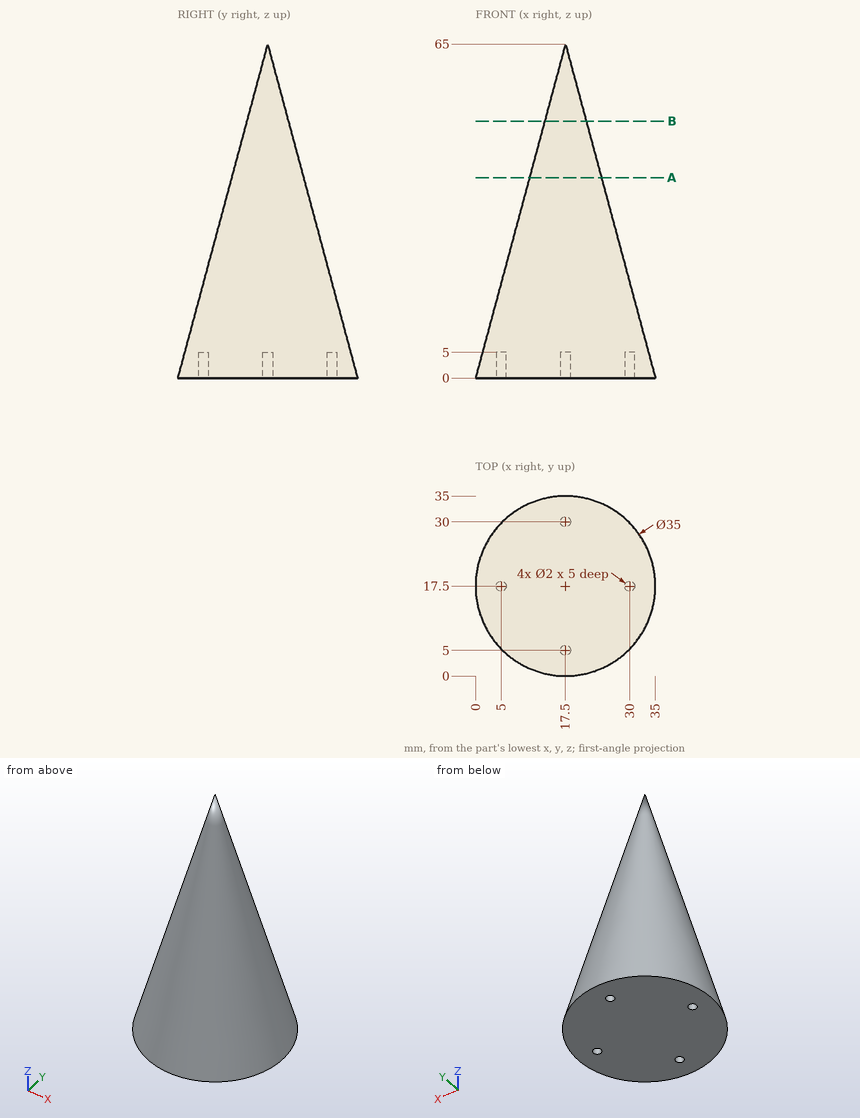
The drawing under review shows one solid part. Ordinate dimensions are in mm from its lowest x, y, z. Round coordinates to 2 decimals unless told otherwise and drop trailing zeros. Loops run counter-clockwise (first coordinate to the right, second up) from the corner with the lowest first, then second, coordinate; pieces in that order, holes last. Notation, with made-up numbers: (87.25, 2.25) - (110.25, 2.25) arc R36 cw to (110.25, 38.25) - close; hole circle Ø4 at (-21, -37). An arc over 180 degrees is marked (long way). One line per item, written item: value. Start each with the question number.
1) To check wall thickness, follow L1, parallel to X at y = 17.5, z = 3.1; L2, parallel to Y at x = 17.5, z = 2.3; L3, parallel to Y at x = 30, z = 3. State the ranges of each line that lie inside material, in increasing order. Write a range as from..to.
2) Consider section A-A on z = 39. Give the boundary of the cut face in (x, y).
3) Consider section B-B on z = 50. Give the boundary of the cut face in (x, y), then the cut area to 3 significant figures.
4) Insertion check: pin 1 Ø5 at (x, z) = (24, 31) entering from +Y; pin 2 Ø0.6 at (x, y) = (5, 17.5) entering from -Z; pin 3 Ø6 at (y, z) = (19.5, 34.5) entering from -X. Each pin has a flat end and moves straight along its axis. Give the tip position at first contact, or say it passes through.
Reported:
1. L1: x = 0.83..4, 6..29, 31..34.17
1. L2: y = 0.62..4, 6..29, 31..34.38
1. L3: y = 6.44..16.5, 18.5..28.56
2. outline: circle Ø14 at (17.5, 17.5)
3. outline: circle Ø8.08 at (17.5, 17.5)
3. area: 51.2 mm^2
4. pin 1: stops at y = 25.94
4. pin 2: stops at z = 5
4. pin 3: stops at x = 8.58
